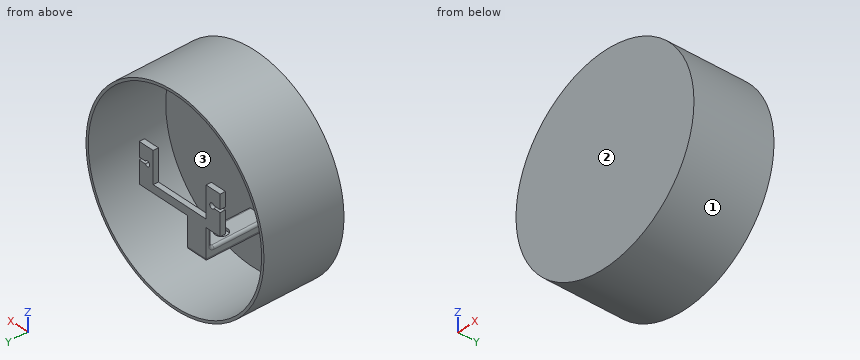
```python
from build123d import *

# Parameters (mm, degrees)
BOSS_EXTRUDE1_DEPTH = 2
SKETCH3_W           = 8
SKETCH3_H           = 13.374853929
BOSS_EXTRUDE2_DEPTH = 4
FILLET1_R           = 1
SKETCH4_R           = 2.35
SKETCH4_R_2         = 0.6
CUT_EXTRUDE1_DEPTH  = 2
SKETCH4_4_R         = 0.6
CUT_EXTRUDE2_DEPTH  = 4
CUT_EXTRUDE3_START  = -4
SKETCH4_5_R         = 2.35
SKETCH4_5_R_2       = 0.6
CUT_EXTRUDE3_DEPTH  = 1
BOSS_EXTRUDE3_START = 10
SKETCH6_R           = 37.280765685
BOSS_EXTRUDE3_DEPTH = 1
EXTRUDE_THIN1_START = 11
SKETCH6_2_R         = 38.280765685
SKETCH6_2_R_2       = 37.280765685
EXTRUDE_THIN1_DEPTH = 30.684854
BOSS_EXTRUDE4_DEPTH = 10


with BuildPart() as part:
    # Sketch1 → Boss-Extrude1 (new body)
    with BuildSketch(Plane(origin=(0, 0, 0), x_dir=(1, 0, 0), z_dir=(0, 1, 0))):
        with BuildLine():
            Line((-11.4, -6), (-17.4, -6))
            Line((-17.4, -6), (-17.4, -0.5))
            Line((-17.4, -0.5), (-14.766025404, -0.5))
            ThreePointArc((-14.766025404, -0.5), (-12.9, 0), (-14.766025404, 0.5))
            Line((-14.766025404, 0.5), (-17.4, 0.5))
            Line((-17.4, 0.5), (-17.4, 9))
            Line((-17.4, 9), (-11.4, 9))
            Line((-11.4, 9), (-11.4, 17))
            Line((-11.4, 17), (-3.4, 17))
            Line((-3.4, 17), (-3.4, 9))
            Line((-3.4, 9), (17.4, 9))
            Line((17.4, 9), (17.4, 0.5))
            Line((17.4, 0.5), (14.766025404, 0.5))
            ThreePointArc((14.766025404, 0.5), (12.9, 0), (14.766025404, -0.5))
            Line((14.766025404, -0.5), (17.4, -0.5))
            Line((17.4, -0.5), (17.4, -6))
            Line((17.4, -6), (11.4, -6))
            Line((11.4, -6), (11.4, 6))
            Line((11.4, 6), (-11.4, 6))
            Line((-11.4, 6), (-11.4, -6))
        make_face()
    extrude(amount=BOSS_EXTRUDE1_DEPTH)

    # Sketch3 → Boss-Extrude2 (add)
    with BuildSketch(Plane(origin=(0, 0, -17), x_dir=(-1, 0, 0), z_dir=(0, 0, -1))):
        with Locations((7.4, -4.687426965)):
            Rectangle(SKETCH3_W, SKETCH3_H)
    extrude(amount=BOSS_EXTRUDE2_DEPTH)

    # Fillet1
    fillet1_edges = [part.edges().sort_by_distance(p)[0] for p in [
        (-11.4, 0, -13),
        (-7.4, 0, -17),
        (-3.4, 0, -13),
        (-3.4, -5.687426964, -17),
        (-11.4, -5.687426964, -17),
        (-3.4, -4.687426964, -21),
        (-11.4, -4.687426964, -21),
        (-7.4, 2, -21),
    ]]
    fillet(fillet1_edges, radius=FILLET1_R)

    # Sketch4 → Cut-Extrude1 (cut)
    with BuildSketch(Plane(origin=(0, 0, -21), x_dir=(-1, 0, 0), z_dir=(0, 0, -1))):
        with Locations((7.4, -7.374853929)):
            Circle(SKETCH4_R)
        with Locations((7.4, -7.374853929)):
            Circle(SKETCH4_R_2, mode=Mode.SUBTRACT)
        with Locations((7.4, -7.374853929)):
            Circle(SKETCH4_R_2)
    extrude(amount=-CUT_EXTRUDE1_DEPTH, mode=Mode.SUBTRACT)

    # Sketch4<4> → Cut-Extrude2 (cut)
    with BuildSketch(Plane(origin=(0, 0, -21), x_dir=(-1, 0, 0), z_dir=(0, 0, -1))):
        with Locations((7.4, -7.374853929)):
            Circle(SKETCH4_4_R)
    extrude(amount=-CUT_EXTRUDE2_DEPTH, mode=Mode.SUBTRACT)

    # Sketch4<5> → Cut-Extrude3 (cut)
    with BuildSketch(Plane(origin=(0, 0, -21), x_dir=(-1, 0, 0), z_dir=(0, 0, -1)).offset(CUT_EXTRUDE3_START)):
        with Locations((7.4, -7.374853929)):
            Circle(SKETCH4_5_R)
        with Locations((7.4, -7.374853929)):
            Circle(SKETCH4_5_R_2, mode=Mode.SUBTRACT)
    extrude(amount=CUT_EXTRUDE3_DEPTH, mode=Mode.SUBTRACT)



with BuildPart() as body_2:
    # Sketch6 → Boss-Extrude3 (new body)
    with BuildSketch(Plane.XZ.offset(11.374853929).offset(BOSS_EXTRUDE3_START)):
        with Locations((-5.05, 0.1)):
            Circle(SKETCH6_R)
    extrude(amount=BOSS_EXTRUDE3_DEPTH)

    # Sketch6<2> → Extrude-Thin1 (add)
    with BuildSketch(Plane.XZ.offset(11.374853929).offset(EXTRUDE_THIN1_START)):
        with Locations((-5.05, 0.1)):
            Circle(SKETCH6_2_R)
        with Locations((-5.05, 0.1)):
            Circle(SKETCH6_2_R_2, mode=Mode.SUBTRACT)
    extrude(amount=-EXTRUDE_THIN1_DEPTH)


with BuildPart() as part_1:
    add(part.part)

    add(body_2.part)  # Boss-Extrude4 merges body 2
    # Sketch7 → Boss-Extrude4 (add)
    with BuildSketch(Plane.XZ.offset(11.374853929)):
        with BuildLine():
            Line((-3.4, -20), (-3.4, -18))
            ThreePointArc((-3.4, -18), (-3.692893219, -17.292893219), (-4.4, -17))
            Line((-4.4, -17), (-10.4, -17))
            ThreePointArc((-10.4, -17), (-11.107106781, -17.292893219), (-11.4, -18))
            Line((-11.4, -18), (-11.4, -20))
            ThreePointArc((-11.4, -20), (-11.107106781, -20.707106781), (-10.4, -21))
            Line((-10.4, -21), (-4.4, -21))
            ThreePointArc((-4.4, -21), (-3.692893219, -20.707106781), (-3.4, -20))
        make_face()
    extrude(amount=BOSS_EXTRUDE4_DEPTH)


solid = part_1.part
```
Could you check a few things on this model? Use its own coordinates, in mm. Face numbers are marked on the shaded views. Round coordinates to 2 decimals unless told otherwise and drop trailing zeros. Write each loop counter-clockwise with the first axis right and the second up, starting at its lowest first coordinate (ties: lowest second). Pieces come first, ordered by that corner, then holes. Notation, with made-up numbers: M 46.25,-15.75 L 86.25,-15.75 A21 cw 86.25,22.25 Z; hole C 63.5,85 d5. An arc over 180 degrees is marked long. Answer in a Markdown table with one row per item. Add a question column.
Q1. If we mould it in two halves opening along X, with no side actions, what happens to the marked faces 1, 2 and 3? For each: +X half, -X half, draft (parallel to the pull), parting line (faces both ways), or undercut.
Q2. Imagine slicing it at B-B (z = -29.5). Please give me the cut outline in (x, y), then the cut area to 3 significant figures.
Q3. Imagine slicing it at A-A (y = -15). Please give me the cut outline in (x, z).
Q4. Will these pins go through, and if not, where does the flat tip stop? pin 1 Ø10 at (x, y) = (-7, -9) entering from -Z; pin 2 Ø10 at (y, z) = (-7.5, -17) entering from +X; pin 3 Ø12 at (y, z) = (-1.5, 19) entering from +X.
Q5. Imagine slicing it at C-C (z = 29). Please give me the cut outline in (x, y).
Q6. If I drill on line 1 (X direction, y = 1, z = 0); line 2 (Y direction, x = -7.4, z = -18.5); line 3 (X direction, y = -3, z = -20), over which ranges is the centre line in solid material (lowest first)? Write a range as from..to.
Values:
| question | item | result |
|---|---|---|
| 1 | face 1 | parting line |
| 1 | face 2 | draft |
| 1 | face 3 | undercut |
| 2 | outline | M -29.32,-22.37 L 19.22,-22.37 L 19.22,8.31 L 17.61,8.31 L 17.61,-21.37 L -27.71,-21.37 L -27.71,8.31 L -29.32,8.31 Z |
| 2 | area | 144 mm^2 |
| 3 | outline | C -5.05,0.1 d76.56; M -11.4,-20 A1 ccw -10.4,-21 L -4.4,-21 A1 ccw -3.4,-20 L -3.4,-18 A1 ccw -4.4,-17 L -10.4,-17 A1 ccw -11.4,-18 Z; hole C -5.05,0.1 d74.56 |
| 4 | pin 1 | z = -38.18 |
| 4 | pin 2 | x = 31.27 |
| 4 | pin 3 | x = 30.99 |
| 5 | outline | M -30.15,-22.37 L 20.05,-22.37 L 20.05,8.31 L 18.5,8.31 L 18.5,-21.37 L -28.6,-21.37 L -28.6,8.31 L -30.15,8.31 Z |
| 6 | line 1 | -43.33..-42.33, -12.9..-11.4, 11.4..12.9, 32.23..33.23 |
| 6 | line 2 | -22.37..-7.97, -6.77..2 |
| 6 | line 3 | -37.63..-36.45, -11.4..-3.4, 26.35..27.53 |
